```python
from build123d import *

# Parameters (mm, degrees)
F0_W          = 33.7692135945
F0_H          = 26.0943928733
F0_W_2        = 4.9886330962
F0_H_2        = 7.2910804302
F0_W_3        = 45.0895689428
F0_H_3        = 28.9724431932
F1_DEPTH      = 25.4
F3_DEPTH      = 45.0895689428
F4_R          = 7.4927788442
F4_R_2        = 13.6349594123
F5_DEPTH      = 35.306
F5_DEPTH_BACK = 22.86
F6_DEPTH      = 25.4
F8_DEPTH      = 22.861
F8_DEPTH_BACK = 35.307
F11_W         = 4.9897357821
F11_H         = 26.1090615085
F11_W_2       = 6.0124509037
F11_H_2       = 26.9668074491
F12_DEPTH     = 5.588


with BuildPart() as f1:
    # F0 (on Top) → F1 (new body)
    with BuildSketch(Plane.XY):
        with Locations((6.3317283057, 27.245614212)):
            Rectangle(F0_W, F0_H)
        with Locations((-2.4943165481, 29.164317064)):
            Rectangle(F0_W_2, F0_H_2, mode=Mode.SUBTRACT)
        with Locations((9.2097842135, 29.164317064)):
            Rectangle(F0_W_2, F0_H_2, mode=Mode.SUBTRACT)
        Polygon((23.2163351029, 14.1984177753), (-10.5528784916, 14.1984177753), (-16.1171220243, 14.1984177753), (-16.1171220243, -28.0130952597), (28.9724469185, -28.0130952597), (28.9724469185, 14.1984177753), align=None)
        with Locations((6.4276624471, -42.4993168563)):
            Rectangle(F0_W_3, F0_H_3)
    extrude(amount=F1_DEPTH)

    # F2 (on face) → F3 (join, through all)
    with BuildSketch(Plane(origin=(-16.1171220243, 0, 0), x_dir=(0, -1, 0), z_dir=(-1, 0, 0))):
        Polygon((56.2180615962, 54.1074834764), (26.784285903, 25.4), (56.9855384529, 25.4), align=None)
    extrude(amount=-F3_DEPTH)

    # F4 (on Right) → F5 (join, two sides)
    with BuildSketch(Plane.YZ) as f5_sk:
        with Locations((-50.2700731158, 39.1415841877)):
            Circle(F4_R)
        with Locations((-47.7757565677, 10.3610064834)):
            Circle(F4_R_2)
    extrude(amount=F5_DEPTH)
    extrude(f5_sk.sketch, amount=-F5_DEPTH_BACK)

    # F0 (on Top) → F6 (join)
    with BuildSketch(Plane.XY):
        with Locations((6.3317283057, 27.245614212)):
            Rectangle(F0_W, F0_H)
        with Locations((-2.4943165481, 29.164317064)):
            Rectangle(F0_W_2, F0_H_2, mode=Mode.SUBTRACT)
        with Locations((9.2097842135, 29.164317064)):
            Rectangle(F0_W_2, F0_H_2, mode=Mode.SUBTRACT)
        Polygon((23.2163351029, 14.1984177753), (-10.5528784916, 14.1984177753), (-16.1171220243, 14.1984177753), (-16.1171220243, -28.0130952597), (28.9724469185, -28.0130952597), (28.9724469185, 14.1984177753), align=None)
        with Locations((6.4276624471, -42.4993168563)):
            Rectangle(F0_W_3, F0_H_3)
    extrude(amount=F6_DEPTH)

    # F7 (on Right) → F8 (cut, two sides)
    with BuildSketch(Plane.YZ) as f8_sk:
        Polygon((-56.4099289477, 54.4912219048), (-56.4099289477, 50.6538152695), (-52.3806512356, 50.6538152695), align=None)
    extrude(amount=-F8_DEPTH, mode=Mode.SUBTRACT)
    extrude(f8_sk.sketch, amount=F8_DEPTH_BACK, mode=Mode.SUBTRACT)

    # F11 (on plane+point) → F12 (join, symmetric)
    with BuildSketch(Plane.XY.offset(12.7)):
        with Locations((-18.6119899154, -6.034891739)):
            Rectangle(F11_W, F11_H)
        with Locations((31.9786723703, -7.1516768159)):
            Rectangle(F11_W_2, F11_H_2)
    extrude(amount=F12_DEPTH, both=True)


solid = f1.part
```
CAD build for the part. Positions are in the model's coordinates, mm. A direction names the side the tool comes from. Round coordinates to 2 decimals unless told otherwise and drop trailing zeros. Loops run counter-clockwise (first coordinate to the right, second up) from the corner with the lowest first, then second, coordinate; pieces in that order, holes last. Notation, with made-up numbers: M -2,37.25 L 55,37.25 A12 cw 55,56.25 Z; hole C 1.25,72 d9. An arc over 180 degrees is marked long. Return JSON: item names as keys, results as strings. Group by question number.
(1) Saw through at D-D, the plane y = 24. List the corners of the cut face in (x, z).
(2) Saw through at B-B, the plane x = -15. List the corners of the cut face in (y, z), and give its area (3 significant figures).
(3) Mould opens along X. For faces 1 (the flat face through (0, 29, 13)), 2 (the flat face through (28.972, -54, 48)), 3 (the flat face through (6, 1, 0)), 4 (the flat face through (9, 25.519, 13)) say: +X half, -X half, draft (parallel to the pull), parting line (faces both ways), or undercut.
(4) Drop flat-ended pins along their axis: P1, Ø1.5, axis at y = 20, z = 26.5, coming from the +X side; P2, Ø2, axis at y = 31, z = 18.5, coming from the +X side; P3, Ø12.5, axis at y = -4, z = 13.5, coming from the -X side; P4, Ø6, axis at y = 28, z = 16.5, coming from the -X side. Give the stop position or say it passes through.
(5) Tool access for faces 5 (the flat face through (6, 40.293, 13)), 6 (the flat face through (9, 32.81, 13)), 7 (the flat face through (-19, 7.02, 13)), 8 (the flat face through (6, 7, 25.4)): list every direction of +Z, -Z, +X, -X, +Y, -Y with a clear straight run to the whole face (end or side of a thin tool).
(6) Saw through at A-A, the plane x = 8. List the corners of the cut face in (y, z), and give its area (3 significant figures).
(7) Saw through at C-C, the plane z = 5.5. List the corners of the cut face in (x, y), and give its area (3 significant figures).
(8) Wall check: probe 1 along X at (y, z) = (29, 22.5); probe 2 along Y at (x, z) = (1, 10.5); probe 3 along Z at (x, y) = (-15, -8). Give the ranges that are in metal, low to high. Write a range as [from, to].
Answer list:
{
 "1": {"outline": "M -10.55,0 L 23.22,0 L 23.22,25.4 L -10.55,25.4 Z"},
 "2": {"outline": "M -56.99,0 L -56.64,0 A13.63 ccw -38.91,0 L 14.2,0 L 14.2,25.4 L -26.78,25.4 L -43.1,41.31 A7.49 ccw -48.28,46.37 L -52.68,50.65 L -56.31,50.65 L -56.51,43.29 A7.49 ccw -56.72,35.33 L -56.99,25.4 L -56.99,20.42 A13.63 ccw -56.99,0.31 Z", "area": "2,350 mm2"},
 "3": {"face 1": "undercut", "face 2": "+X half", "face 3": "draft", "face 4": "undercut"},
 "4": {"P1": "through", "P2": "x = 23.22", "P3": "x = -21.11", "P4": "x = -10.55"},
 "5": {"face 5": "+Z, -Z, +X, -X, +Y", "face 6": "+Z, -Z", "face 7": "+Z, -Z, -X, +Y", "face 8": "+Z, +X, -X, +Y"},
 "6": {"outline": "M -56.99,0 L -56.64,0 A13.63 ccw -38.91,0 L 25.52,0 L 25.52,25.4 L -26.78,25.4 L -43.1,41.31 A7.49 ccw -48.28,46.37 L -52.68,50.65 L -56.31,50.65 L -56.51,43.29 A7.49 ccw -56.72,35.33 L -56.99,25.4 L -56.99,20.42 A13.63 ccw -56.99,0.31 Z; M 32.81,0 L 40.29,0 L 40.29,25.4 L 32.81,25.4 Z", "area": "2,820 mm2"},
 "7": {"outline": "M -22.86,-60.51 L 35.31,-60.51 L 35.31,-35.04 L 28.97,-35.04 L 28.97,14.2 L 23.22,14.2 L 23.22,40.29 L -10.55,40.29 L -10.55,14.2 L -16.12,14.2 L -16.12,-35.04 L -22.86,-35.04 Z; hole M -4.99,25.52 L 0,25.52 L 0,32.81 L -4.99,32.81 Z; hole M 6.72,25.52 L 11.7,25.52 L 11.7,32.81 L 6.72,32.81 Z", "area": "4,510 mm2"},
 "8": {"probe 1": "[-10.55, -4.99], [0, 6.72], [11.7, 23.22]", "probe 2": "[-61.41, 40.29]", "probe 3": "[0, 25.4]"}
}
